CAD build for the part. Positions are in the model's coordinates, mm. Face numbers are marked on the shaded views. A direction names the side the tool comes from. Give positions to 0.01 mm unless a question says otherwise; leave off trailing zeros. Loops run counter-clockwise (first coordinate to the right, second up) from the corner with the lowest first, then second, coordinate; pieces in that order, holes last.
Item 1: Saw through at C-C on z = -15.5. Give the cut face in (x, y), plus the area to 3 significant figures.
Item 2: Saw through at B-B on x = -12.5. Give the cut face in (y, z).
Item 3: Drop flat-ended pins along their axis: P1, Ø15, axis at x = -5, y = 19.5, coming from the +Z side; P2, Ø8, axis at x = -28, z = 37, coming from the +Y side; P3, Ø5.5, axis at x = 34, y = -31.5, coming from the -Z side. Give the stop position or say it passes through.
Item 4: Mould opens along X. For the marked faces 4, 5 and 6 say: released by +X, released by -X, zero draft, split by the parting line, or undercut.
Item 5: Saw through at A-A on y = -1.5. Give the cut face in (x, z).
Item 6: Which spindle directions (+Z, -Z, +X, -X, +Y, -Y) get a long thin tool onto all of the face, cutting with end or side? Do the marked faces 1, 2 and 3. Say none if no direction does.
Item 7: Probe probe 1 along Y at (x, z) = (-24.5, 38.5); probe 2 along Y at (x, z) = (40, -12.5); probe 3 along Z at (x, y) = (35, 34). List the from-to ranges inside material, lowest first.
Item 8: Saw through at D-D on z = 63. Give the cut face in (x, y).
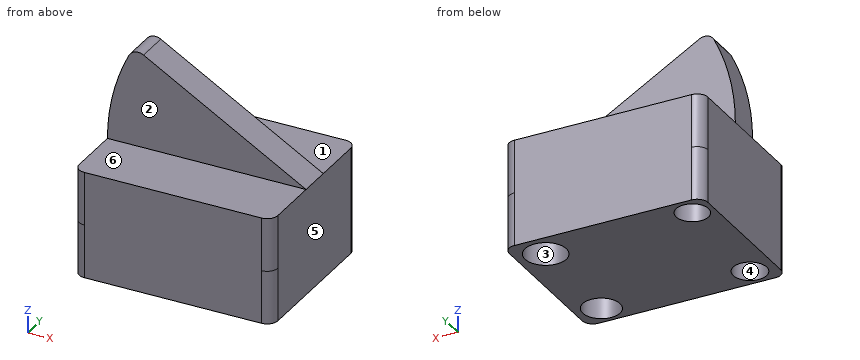
from build123d import *

# Parameters (mm, degrees)
F0_W     = 94.5846885443
F0_H     = 28.4219961613
F0_H_2   = 24.2285877466
F0_H_3   = 23.2967082411
F1_DEPTH = 25.4
F2_W     = 94.5846885443
F2_H     = 15.5447232537
F3_ANGLE = 30
F4_R     = 5.08
F5_R     = 5.08
F6_R     = 5.08
F7_R     = 7.7354958654
F7_R_2   = 9.827935595
F7_R_3   = 7.966520615
F7_R_4   = 8.8977236071
F8_DEPTH = 25.4


with BuildPart() as f1:
    # F0 (on Top) → F1 (new body)
    with BuildSketch(Plane.XY):
        with Locations((0, 0.4659397528)):
            Rectangle(F0_W, F0_H)
        with Locations((0, -25.8593522012)):
            Rectangle(F0_W, F0_H_2)
        with Locations((0, 26.325291954)):
            Rectangle(F0_W, F0_H_3)
    extrude(amount=F1_DEPTH)

    # F2 (on face) → F3 (revolve)
    with BuildSketch(Plane.XY.offset(25.4)):
        with Locations((0, 0.3310537431)):
            Rectangle(F2_W, F2_H)
    revolve(axis=Axis((47.2923442721, 0.3310537431, 25.4), (0, 1, 0)), revolution_arc=F3_ANGLE)

    # F4
    f4_edges = [f1.edges().sort_by_distance(p)[0] for p in [
        (-47.292344, -37.973646, 12.7),
        (47.292344, -37.973646, 12.7),
    ]]
    fillet(f4_edges, radius=F4_R)

    # F5
    f5_edges = [f1.edges().sort_by_distance(p)[0] for p in [
        (47.292344, 37.973646, 12.7),
    ]]
    fillet(f5_edges, radius=F5_R)

    # F6
    f6_edges = [f1.edges().sort_by_distance(p)[0] for p in [
        (-47.292344, 37.973646, 12.7),
        (-34.620399, 0.331054, 72.692344),
    ]]
    fillet(f6_edges, radius=F6_R)

    # F7 (on face) → F8 (join)
    with BuildSketch(Plane(origin=(0, 0, 0), x_dir=(1, 0, 0), z_dir=(0, 0, -1))):
        with BuildLine():
            ThreePointArc((-47.2923442721, -32.8936460745), (-45.8044467206, -36.485748523), (-42.2123442721, -37.9736460745))
            Line((-42.2123442721, -37.9736460745), (42.2123442721, -37.9736460745))
            ThreePointArc((42.2123442721, -37.9736460745), (45.8044467206, -36.485748523), (47.2923442721, -32.8936460745))
            Line((47.2923442721, -32.8936460745), (47.2923442721, 32.8936460745))
            ThreePointArc((47.2923442721, 32.8936460745), (45.8044467206, 36.485748523), (42.2123442721, 37.9736460745))
            Line((42.2123442721, 37.9736460745), (-42.2123442721, 37.9736460745))
            ThreePointArc((-42.2123442721, 37.9736460745), (-45.8044467206, 36.485748523), (-47.2923442721, 32.8936460745))
            Line((-47.2923442721, 32.8936460745), (-47.2923442721, -32.8936460745))
        make_face()
        with Locations((-37.3279750347, -27.9809720814)):
            Circle(F7_R, mode=Mode.SUBTRACT)
        with Locations((33.9089371264, -25.3520905972)):
            Circle(F7_R_2, mode=Mode.SUBTRACT)
        with Locations((-35.1918712258, 28.0274003744)):
            Circle(F7_R_3, mode=Mode.SUBTRACT)
        with Locations((35.1046472788, 27.1290969104)):
            Circle(F7_R_4, mode=Mode.SUBTRACT)
    extrude(amount=F8_DEPTH)


solid = f1.part
Results below:
1. outline: (-47.29, -32.89) arc R5.08 ccw to (-42.21, -37.97) - (42.21, -37.97) arc R5.08 ccw to (47.29, -32.89) - (47.29, 32.89) arc R5.08 ccw to (42.21, 37.97) - (-42.21, 37.97) arc R5.08 ccw to (-47.29, 32.89) - close; hole circle Ø15.47 at (-37.33, 27.98); hole circle Ø15.93 at (-35.19, -28.03); hole circle Ø19.66 at (33.91, 25.35); hole circle Ø17.8 at (35.1, -27.13)
1. area: 6,220 mm2
2. outline: (-37.97, -25.4) - (37.97, -25.4) - (37.97, 25.4) - (8.1, 25.4) - (8.1, 59.92) - (-7.44, 59.92) - (-7.44, 25.4) - (-37.97, 25.4) - close
3. P1: stops at z = 25.4
3. P2: stops at y = 8.1
3. P3: stops at z = 0
4. face 4: undercut
4. face 5: released by +X
4. face 6: zero draft
5. outline: (-47.29, -25.4) - (47.29, -25.4) - (47.29, 25.4) - (-30.1, 70.08) arc R5.08 ccw to (-37.17, 67.97) arc R94.58 ccw to (-47.29, 25.4) - close
6. face 1: +Z, +X, -X, +Y
6. face 2: +Z, +X, -X, -Y
6. face 3: -Z
7. probe 1: y = -7.44 to 8.1
7. probe 2: y = -37.97 to -34.56, -19.7 to 17.64, 33.06 to 37.97
7. probe 3: z = 0 to 25.4
8. outline: (-39.5, -7.44) - (-17.83, -7.44) - (-17.83, 8.1) - (-39.5, 8.1) - close
